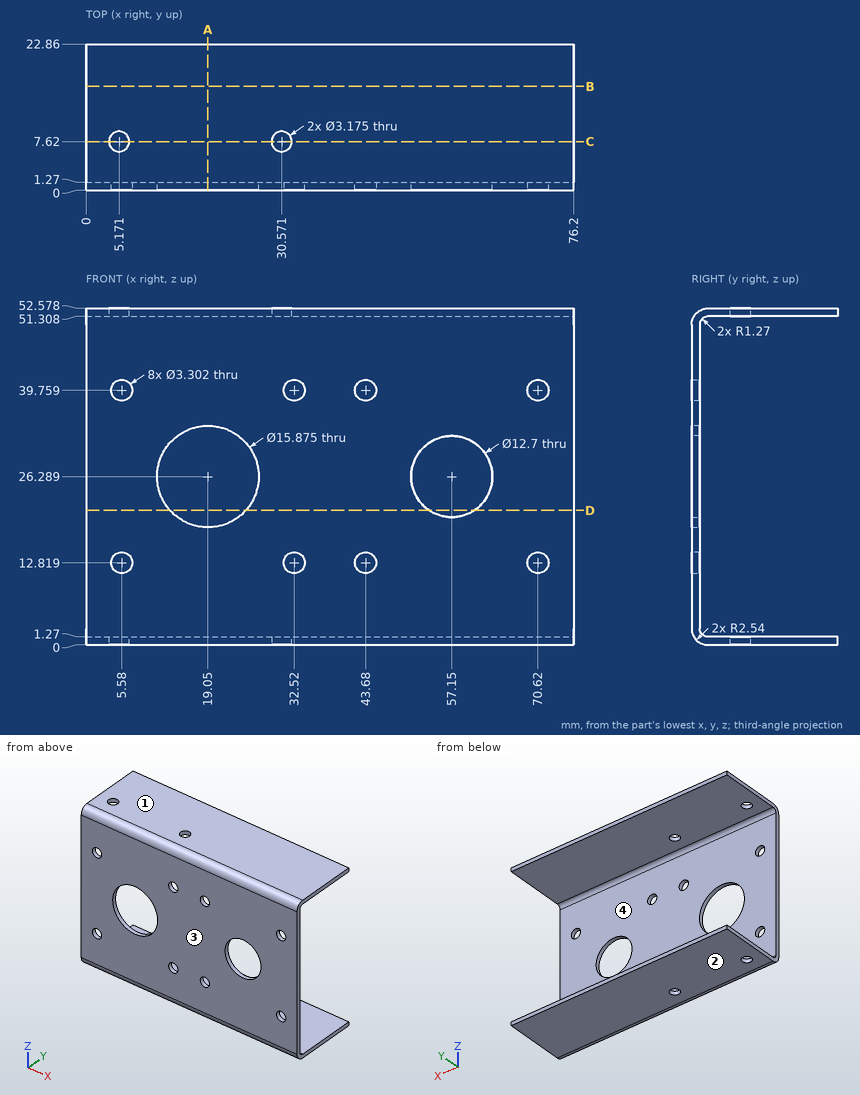
Verification items for this drawing (mm, ordinates from the low corner). Round coordinates to 2 decimals unless told otherwise and drop trailing zeros. Loops run counter-clockwise (first coordinate to the right, second up) from the corner with the lowest first, then second, coordinate; pieces in that order, holes last. Notation, with made-up numbers: (3.5, 2.5) -> (8.5, 2.5) arc R30 cw to (8.5, 40.5) -> close; hole circle Ø1 at (12, 49). An arc over 180 degrees is marked (long way). Answer in a Markdown table with one row per item.
Q1. Thickness scan on L1, parallel to Z at x = 71, y = 9.5; L2, parallel to X at y = 7.62, z = 0.3; L3, parallel to Y at x = 8, z = 42. Record the ranges inside material, lowest first.
Data:
| item | result |
|---|---|
| L1 | z = 0 to 1.27, 51.31 to 52.58 |
| L2 | x = 0 to 3.58, 6.76 to 28.98, 32.16 to 76.2 |
| L3 | y = 0 to 1.27 |
Q2. Release check for a two-part mould opening along Z. For the marked faces 1, 2, 3 and 4 record: released by +Z, released by -Z, zero draft, split by the parting line, or undercut.
Data:
| item | result |
|---|---|
| face 1 | released by +Z |
| face 2 | released by -Z |
| face 3 | zero draft |
| face 4 | undercut |
Q3. Sectioned sample at B-B on y = 16.25. Enter the section's corners in (x, z).
Data:
| item | result |
|---|---|
| outline | (0, 0) -> (76.2, 0) -> (76.2, 1.27) -> (0, 1.27) -> close; (0, 51.31) -> (76.2, 51.31) -> (76.2, 52.58) -> (0, 52.58) -> close |
Q4. Sectioned sample at C-C on y = 7.62. Enter the section's corners in (x, z).
Data:
| item | result |
|---|---|
| outline | (0, 0) -> (3.58, 0) -> (3.58, 1.27) -> (0, 1.27) -> close; (0, 51.31) -> (3.58, 51.31) -> (3.58, 52.58) -> (0, 52.58) -> close; (6.76, 0) -> (28.98, 0) -> (28.98, 1.27) -> (6.76, 1.27) -> close; (6.76, 51.31) -> (28.98, 51.31) -> (28.98, 52.58) -> (6.76, 52.58) -> close; (32.16, 0) -> (76.2, 0) -> (76.2, 1.27) -> (32.16, 1.27) -> close; (32.16, 51.31) -> (76.2, 51.31) -> (76.2, 52.58) -> (32.16, 52.58) -> close |
Q5. Go/stop test with a flat-tipped pin: P1, Ø12, axis at x = 50.5, z = 39, coming from the +Y side. Record where the tip stops, or that it passes through.
Data:
| item | result |
|---|---|
| P1 | stops at y = 1.27 |
Q6. Sectioned sample at D-D on z = 21. Enter the section's corners in (x, y) (1 decimal).
Data:
| item | result |
|---|---|
| outline | (0, 0) -> (13.1, 0) -> (13.1, 1.3) -> (0, 1.3) -> close; (25, 0) -> (53.6, 0) -> (53.6, 1.3) -> (25, 1.3) -> close; (60.7, 0) -> (76.2, 0) -> (76.2, 1.3) -> (60.7, 1.3) -> close |
Q7. Sectioned sample at A-A on x = 19.05. Enter the section's corners in (y, z).
Data:
| item | result |
|---|---|
| outline | (0, 2.54) arc R2.54 ccw to (2.54, 0) -> (22.86, 0) -> (22.86, 1.27) -> (2.54, 1.27) arc R1.27 cw to (1.27, 2.54) -> (1.27, 18.35) -> (0, 18.35) -> close; (0, 34.23) -> (1.27, 34.23) -> (1.27, 50.04) arc R1.27 cw to (2.54, 51.31) -> (22.86, 51.31) -> (22.86, 52.58) -> (2.54, 52.58) arc R2.54 ccw to (0, 50.04) -> close |
